Input: dimensioned drawing with shaded views. Units: mm. Origin: part minimum x, y, z. Round coordinates to 2 decimals unless told otherwise and drop trailing zeros. Write each loop counter-clockwise with the first axis right and the second up, starting at its lowest first coordinate (ties: lowest second). Pieces come first, ordered by that corner, then holes. Notation, with made-up numbers: (30, 80.5) -> (52, 80.5) arc R27 cw to (52, 117.5) -> close; hole circle Ø2 at (-4.5, 42.5). An arc over 180 degrees is marked (long way). One line per item, written item: value. Start each with the question number.
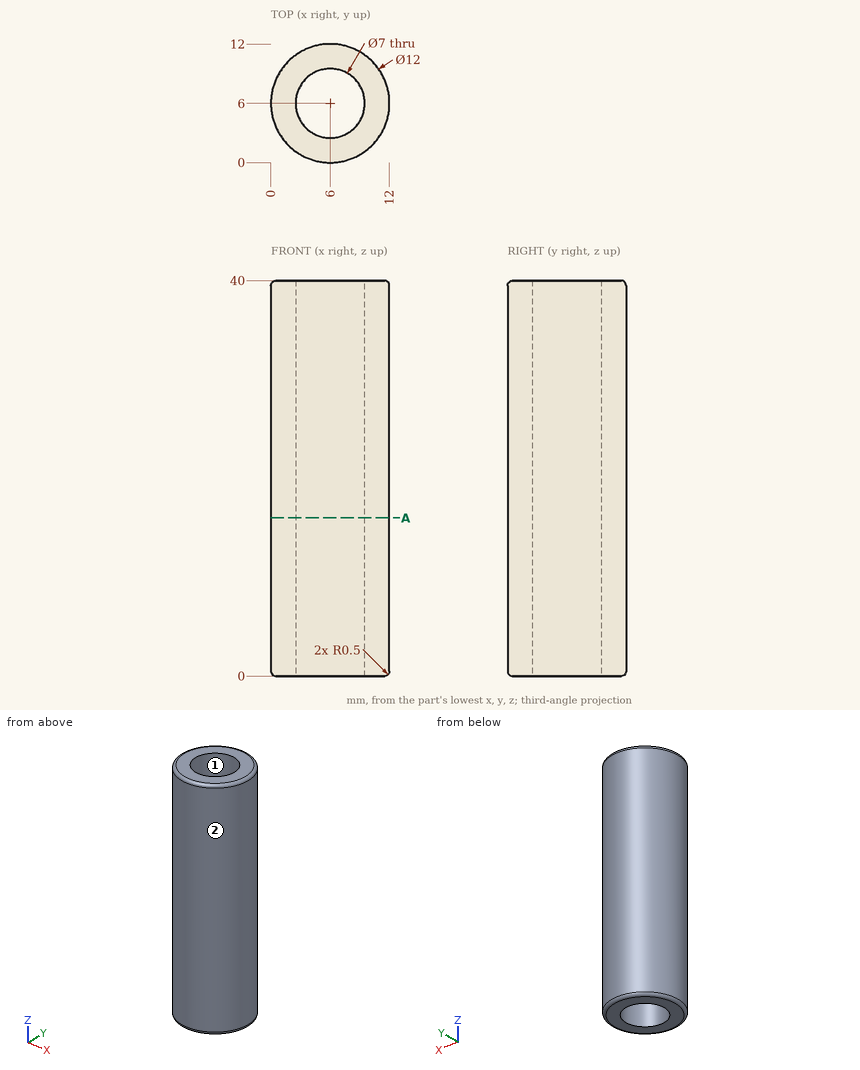
(1) Line query: probe 1 along Y at (x, z) = (6, 19.5); probe 2 along Y at (x, z) = (7, 21.5); probe 3 along X at (y, z) = (7.75, 32). Output: solid intervals per line, ascending.
(2) Section query A-A (z = 16). Output: boundary loops of the cut face in (x, y), and give its area (3 significant figures).
(3) Pin query (flat end, axial travel): pin 1 (5 mm diameter, centred on y = 8.5, z = 24.5, fed in from -X); pin 2 (4 mm diameter, centred on y = 2, z = 32.5, fed in from -X). Return the tip coordinate at first contact, or that it passes through.
(4) Pull-direction query (X, two-part tool) for the marked faces 1 and 2; classes: pulls with the +X half, pulls with the -X half, needs draft (parallel to the pull), parting line crosses it, or undercut.
Results list:
1. probe 1: y = 0 to 2.5, 9.5 to 12
1. probe 2: y = 0.08 to 2.65, 9.35 to 11.92
1. probe 3: x = 0.26 to 2.97, 9.03 to 11.74
2. outline: circle Ø12 at (6, 6); hole circle Ø7 at (6, 6)
2. area: 74.6 mm^2
3. pin 1: stops at x = 0
3. pin 2: stops at x = 0.34
4. face 1: undercut
4. face 2: parting line crosses it
